For this review, use the dimensioned drawing (mm, ordinates from the lowest corner) and the shaded views. A direction names the side the tool comes from. Round coordinates to 2 decimals unless told otherwise and drop trailing zeros. Write each loop counter-clockwise with the first axis right and the second up, starting at its lowest first coordinate (ties: lowest second). Pieces come first, ordered by that corner, then holes.
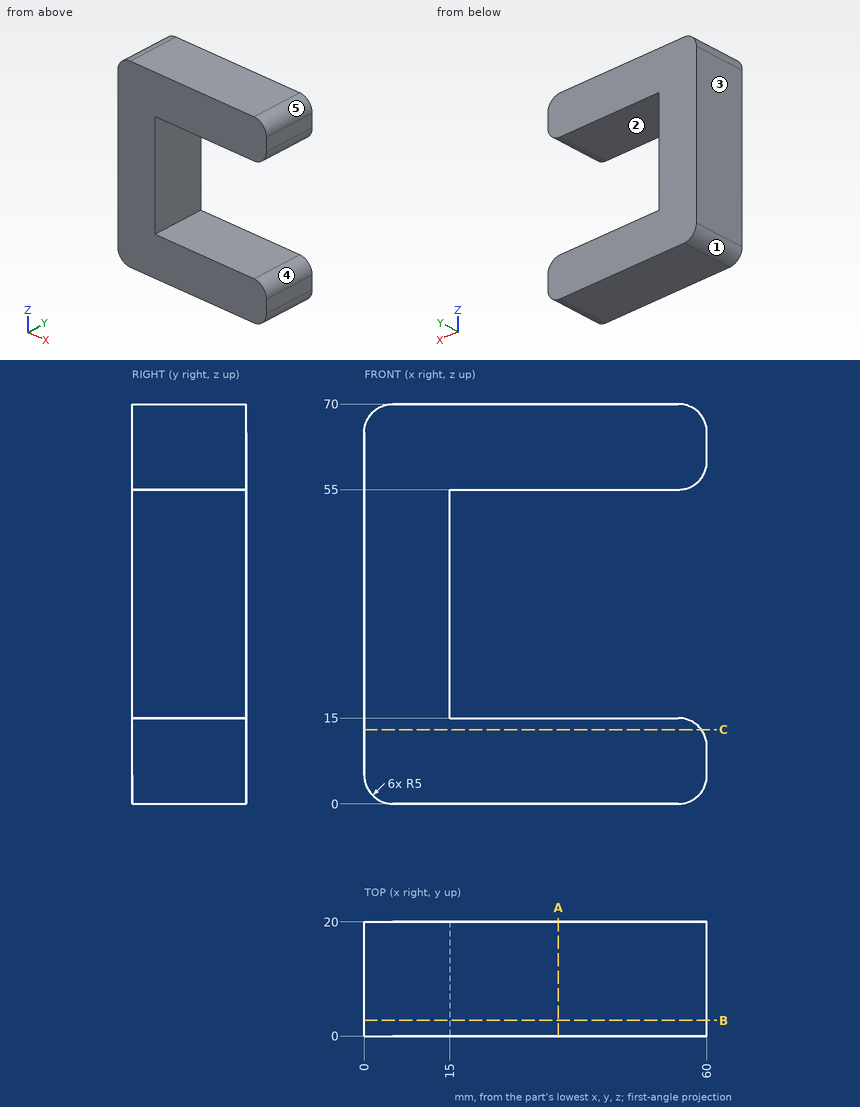
(1) Mouldability with a two-part tool opening along Z and no side actions: class the marked faces 3, 4 and 5 as pulls with the +Z half, pulls with the -Z half, needs draft (parallel to the pull), parting line crosses it, or undercut.
Geometry check:
face 3: needs draft
face 4: undercut
face 5: pulls with the +Z half
(2) For pin 1 Ø3 at (y, z) = (12.5, 50) entering from +X, flat-tipped, find the tip position at first contact; note if it passes through.
Geometry check:
pin 1: stops at x = 15
(3) We need section B-B, the plane y = 2.75. Give the boundary of the cut face in (x, z), and give its area (3 significant figures).
Geometry check:
outline: (0, 5) arc R5 ccw to (5, 0) - (55, 0) arc R5 ccw to (60, 5) - (60, 10) arc R5 ccw to (55, 15) - (15, 15) - (15, 55) - (55, 55) arc R5 ccw to (60, 60) - (60, 65) arc R5 ccw to (55, 70) - (5, 70) arc R5 ccw to (0, 65) - close
area: 2,370 mm2
(4) We need section C-C, the plane z = 13. Give the boundary of the cut face in (x, y), and give its area (3 significant figures).
Geometry check:
outline: (0, 0) - (59, 0) - (59, 20) - (0, 20) - close
area: 1,180 mm2
(5) We need section A-A, the plane x = 34. Give the boundary of the cut face in (y, z), and give its area (3 significant figures).
Geometry check:
outline: (0, 0) - (20, 0) - (20, 15) - (0, 15) - close; (0, 55) - (20, 55) - (20, 70) - (0, 70) - close
area: 600 mm2
(6) For line 1 along Z through (x, y) = (40.5, 15.5); line 2 along X through (y, z) = (15.5, 49); line 3 along Z through (x, y) = (56.5, 14.25), list the stretches that pass through material, from the lowest coordinate up.
Geometry check:
line 1: z = 0 to 15, 55 to 70
line 2: x = 0 to 15
line 3: z = 0.23 to 14.77, 55.23 to 69.77
(7) For the marked faces 1 and 2, list the 3-axis set-ups (+Z, -Z, +X, -X, +Y, -Y) from which the entire face can be reached by the end or side of a thin tool; tool diameter is ignored.
Geometry check:
face 1: -Z, -X, +Y, -Y
face 2: +X, +Y, -Y
